from build123d import *

# Parameters (mm, degrees)
SKETCH1_W           = 169.8625
SKETCH1_H           = 95.25
BOSS_EXTRUDE1_DEPTH = 1.5494
SKETCH2_W           = 15.748
SKETCH2_H           = 18.6436
BOSS_EXTRUDE2_DEPTH = 13.4112
SKETCH3_R           = 4.4704
BOSS_EXTRUDE3_DEPTH = 13.843
SKETCH4_R           = 2.95275
BOSS_EXTRUDE4_DEPTH = 17.1704
SKETCH5_W           = 53.34
SKETCH5_H           = 68.58
BOSS_EXTRUDE5_DEPTH = 14.478
SKETCH6_R           = 2.95275
CUT_EXTRUDE1_DEPTH  = 14.478


with BuildPart() as part:
    # Sketch1 → Boss-Extrude1 (new body)
    with BuildSketch(Plane(origin=(0, 0, 0), x_dir=(1, 0, 0), z_dir=(0, 1, 0))):
        with Locations((84.93125, 47.625)):
            Rectangle(SKETCH1_W, SKETCH1_H)
    extrude(amount=BOSS_EXTRUDE1_DEPTH)

    # Sketch2 → Boss-Extrude2 (add)
    with BuildSketch(Plane(origin=(0, 1.5494, 0), x_dir=(1, 0, 0), z_dir=(0, 1, 0))):
        with Locations((116.2685, 84.2264)):
            Rectangle(SKETCH2_W, SKETCH2_H)
    extrude(amount=BOSS_EXTRUDE2_DEPTH)

    # Sketch3 → Boss-Extrude3 (add)
    with BuildSketch(Plane(origin=(0, 1.5494, 0), x_dir=(1, 0, 0), z_dir=(0, 1, 0))):
        with Locations((60.325, 79.629)):
            Circle(SKETCH3_R)
        with Locations((60.325, 39.751)):
            Circle(SKETCH3_R)
    extrude(amount=BOSS_EXTRUDE3_DEPTH)

    # Sketch4 → Boss-Extrude4 (add)
    with BuildSketch(Plane(origin=(0, 1.5494, 0), x_dir=(1, 0, 0), z_dir=(0, 1, 0))):
        with Locations((48.6791, 15.24)):
            Circle(SKETCH4_R)
        with Locations((74.0791, 15.24)):
            Circle(SKETCH4_R)
    extrude(amount=BOSS_EXTRUDE4_DEPTH)

    # Sketch5 → Boss-Extrude5 (add)
    with BuildSketch(Plane(origin=(0, 0, 0), x_dir=(-1, 0, 0), z_dir=(0, -1, 0))):
        with Locations((-123.6345, 35.3822)):
            Rectangle(SKETCH5_W, SKETCH5_H)
    extrude(amount=BOSS_EXTRUDE5_DEPTH)

    # Sketch6 → Cut-Extrude1 (cut)
    with BuildSketch(Plane(origin=(0, 1.5494, 0), x_dir=(1, 0, 0), z_dir=(0, 1, 0))):
        with Locations((9.81075, 85.08365)):
            Circle(SKETCH6_R)
        with Locations((160.05175, 85.08365)):
            Circle(SKETCH6_R)
        with Locations((160.05175, 9.96315)):
            Circle(SKETCH6_R)
        with Locations((9.81075, 9.96315)):
            Circle(SKETCH6_R)
    extrude(amount=-CUT_EXTRUDE1_DEPTH, mode=Mode.SUBTRACT)


solid = part.part
Model file for the job. Use its own axes, mm. A direction names the side the tool comes from. Give positions to 0.01 mm unless a question says otherwise; leave off trailing zeros. Order: outer loops, then holes, each group sorted by start corner. A loop starts at its lowest first (then second) coordinate and runs counter-clockwise, first axis right, second up. Notation, with made-up numbers: (-19, 49.5) - (-10, 49.5) arc R18 ccw to (-10, 59.5) - close; hole circle Ø9 at (7, 64.25). An arc over 180 degrees is marked (long way). Write item = value, one per line. Start each with the question number.
1. Which spindle directions (+Z, -Z, +X, -X, +Y, -Y) get a long thin tool onto all of the face, cutting with end or side? Do faces 1 (the flat face through (124.142, 8, -84)), 2 (the flat face through (150.305, -7, -35)), 3 (the flat face through (116, 8, -93.548)). Say none if no direction does.
2. Cut at B-B, the plane x = 148. List the corners of the cut face in (y, z).
3. Drop flat-ended pins along their axis: P1, Ø6, axis at y = 5, z = -25, coming from the +X side; P2, Ø10, axis at y = 11, z = -79.5, coming from the +X side; P3, Ø12, axis at y = 10, z = -22, coming from the +X side; P4, Ø9.5, axis at x = 160.05, z = -85.08, coming from the -Y side. Give the stop position or say it passes through.
4. Cut at D-D, the plane y = -4. List the corners of the cut face in (x, z), and give its area (3 significant figures).
5. Cut at A-A, the plane y = 10.5. List the corners of the cut face in (x, z) (1 decimal).
6. Cut at C-C, the plane z = -15.24. List the corners of the cut face in (x, y), and give its area (3 significant figures).
7. Probe line 1 along X through (y, z) = (1, -11.5); line 2 along Y through (x, z) = (73.5, -26); line 3 along Y through (x, z) = (130, -28). List the from-to ranges inside material, lowest first.
8. Two-plate mould, pull along Z, no slides. Class faces 4 (the flat face through (124, -7, -1.092)), 5 (the cylindrical face through (71.13, 10.01, -15.37)), 6 (the cylindrical face through (56.777, 8.374, -76.909)): pulls with the +Z half, pulls with the -Z half, needs draft (parallel to the pull), parting line crosses it, or undercut.
Taken from the geometry:
q1.face_1 = +Z, -Z, +X, +Y
q1.face_2 = +Z, -Z, +X, -Y
q1.face_3 = -Z, +X, -X, +Y
q2.outline = (-14.48, -69.67) - (0, -69.67) - (0, -95.25) - (1.55, -95.25) - (1.55, 0) - (0, 0) - (0, -1.09) - (-14.48, -1.09) - close
q3.P1 = through
q3.P2 = 124.14
q3.P3 = 76.93
q3.P4 = 0
q4.outline = (96.96, -69.67) - (150.3, -69.67) - (150.3, -1.09) - (96.96, -1.09) - close
q4.area = 3,660 mm²
q5.outline = circle Ø5.9 at (48.7, -15.2); circle Ø8.9 at (60.3, -79.6); circle Ø8.9 at (60.3, -39.8); circle Ø5.9 at (74.1, -15.2); (108.4, -93.5) - (124.1, -93.5) - (124.1, -74.9) - (108.4, -74.9) - close
q6.outline = (0, 0) - (96.96, 0) - (96.96, -14.48) - (150.3, -14.48) - (150.3, 0) - (169.86, 0) - (169.86, 1.55) - (77.03, 1.55) - (77.03, 18.72) - (71.13, 18.72) - (71.13, 1.55) - (51.63, 1.55) - (51.63, 18.72) - (45.73, 18.72) - (45.73, 1.55) - (0, 1.55) - close
q6.area = 1,240 mm²
q7.line_1 = 0 to 7.29, 12.33 to 157.53, 162.57 to 169.86
q7.line_2 = 0 to 1.55
q7.line_3 = -14.48 to 1.55
q8.face_4 = pulls with the +Z half
q8.face_5 = parting line crosses it
q8.face_6 = undercut
